Can you work these out from the drawing? Everything is in mm from the part's minimum corner. A direction names the side the tool comes from. Give positions to 0.01 mm unless a question says otherwise; leave off trailing zeros. Order: outer loops, then holes, each group sorted by start corner. A loop starts at its lowest first (then second) coordinate and runs counter-clockwise, first axis right, second up. Notation, with made-up numbers: (82.5, 19) - (98.5, 19) arc R13 ccw to (98.5, 41) - close; hole circle Ø8 at (6, 54). An arc over 180 degrees is marked (long way). One line per question, with ' | ' between items.
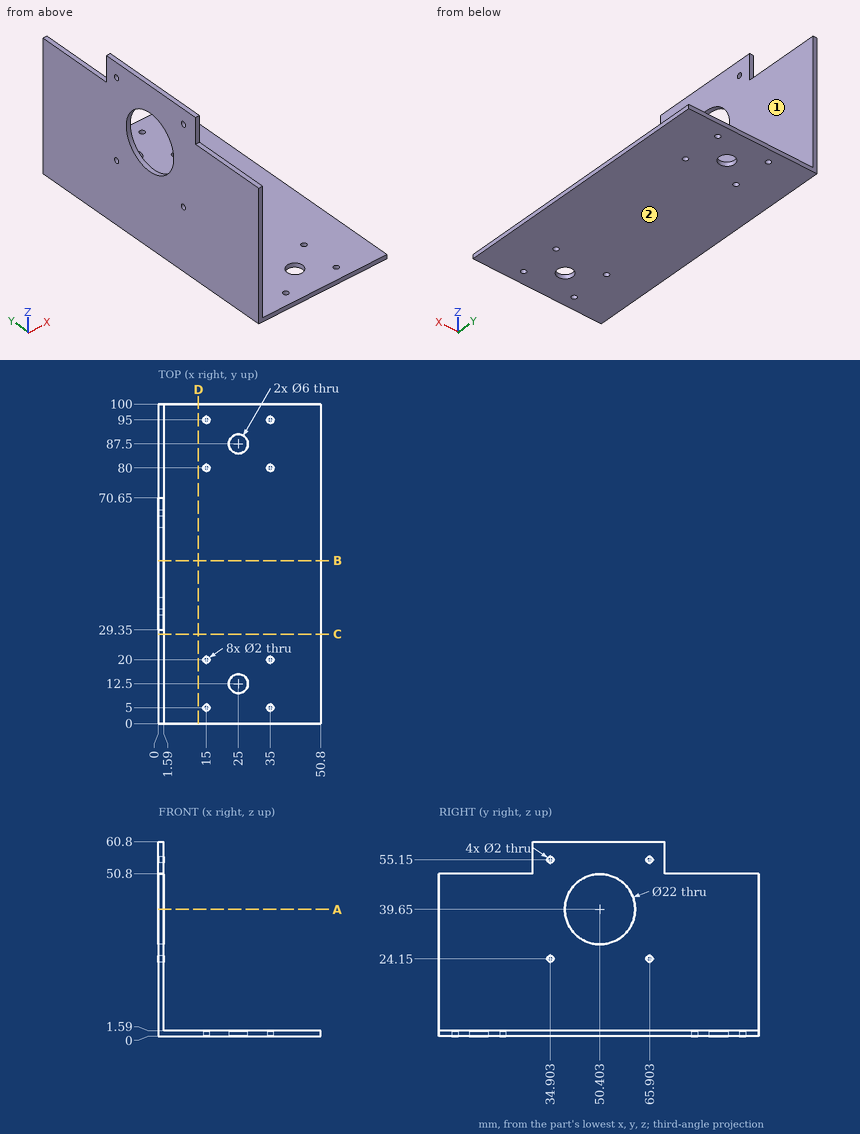
1) Please list where these lines run through material, in increasing order: L1, parallel to Y at x = 1.3, z = 24.15; L2, parallel to Y at x = 0.7, z = 55.15; L3, parallel to X at y = 20, z = 0.5.
Model answer:
L1: y = 0 to 33.9, 35.9 to 64.9, 66.9 to 100 | L2: y = 29.35 to 33.9, 35.9 to 64.9, 66.9 to 70.65 | L3: x = 0 to 14, 16 to 34, 36 to 50.8
2) I want a section at B-B (y = 51). List the corners of the cut face in (x, z) for me, plus the area to 3 significant figures.
Model answer:
outline: (0, 0) - (50.8, 0) - (50.8, 1.59) - (1.59, 1.59) - (1.59, 28.67) - (0, 28.67) - close; (0, 50.63) - (1.59, 50.63) - (1.59, 60.8) - (0, 60.8) - close | area: 140 mm2
3) On a 3-axis mill with a long thin cutter (end or side, diameter ignored), from which of +Z, -Z, +X, -X, +Y, -Y can I reach the whole of each face in a straight line? I mean the marked faces 1 and 2. Say none if no direction works.
Model answer:
face 1: +Z, +X, +Y, -Y | face 2: -Z, +X, -X, +Y, -Y
4) I want a section at C-C (y = 28). List the corners of the cut face in (x, z) for me.
Model answer:
outline: (0, 0) - (50.8, 0) - (50.8, 1.59) - (1.59, 1.59) - (1.59, 50.8) - (0, 50.8) - close
5) I'm going to push flat-ended pins straight in: P1, Ø1.8, axis at y = 34.9, z = 55.15, coming from the +X side; P2, Ø2.5, axis at x = 35, y = 95, coming from the +Z side; P3, Ø10, axis at y = 18, z = 23, coming from the +X side; P4, Ø0.8, axis at x = 0.5, y = 83, coming from the +Z side. Where does each tip first touch, or does it pass through?
Model answer:
P1: passes through | P2: stops at z = 1.59 | P3: stops at x = 1.59 | P4: stops at z = 50.8
6) I want a section at A-A (z = 39.65). List the corners of the cut face in (x, y) for me, plus the area to 3 significant figures.
Model answer:
outline: (0, 0) - (1.59, 0) - (1.59, 39.4) - (0, 39.4) - close; (0, 61.4) - (1.59, 61.4) - (1.59, 100) - (0, 100) - close | area: 124 mm2
7) I want a section at D-D (x = 12.5). List the corners of the cut face in (y, z) for me, plus the area to 3 significant figures.
Model answer:
outline: (0, 0) - (100, 0) - (100, 1.59) - (0, 1.59) - close | area: 159 mm2
